The figure shows three views and two pictorial views of one solid part (mm, origin at its lowest corner). Answer the questions. A direction names the side the tool comes from. Give positions to 0.01 mm unless a question says otherwise; leave off trailing zeros. Order: outer loops, then holes, each group sorted by start corner. A loop starts at its lowest first (then second) coordinate and runs counter-clockwise, first axis right, second up. Notation, with made-up numbers: (37.5, 78) - (44.5, 78) arc R27 ccw to (44.5, 96) - close; hole circle Ø1 at (23, 56.25). An arc over 180 degrees is marked (long way). Answer as CSV lines item,"result". Start each with the question number.
1. Section A-A on y = 61 is taken. Give the vertices of the cut face in (x, z).
2. Consider line 1 along X through (y, z) = (61, 1.75); line 2 along Y through (x, z) = (31, 12); line 3 along Z through (x, y) = (41.5, 62). Determine where each line is inside the solid, lowest interval first. Write a range as [from, to].
3. Which of the six approach directions +Z, -Z, +X, -X, +Y, -Y give full straight-line access (tool end or side, diameter ignored) to the marked faces 1, 2 and 3?
4. Section D-D on y = 47.5 is taken. Give the vertices of the cut face in (x, z).
5. Section C-C on x = 56 is taken. Give the vertices of the cut face in (y, z), and give its area (3 significant figures).
6. Section B-B on z = 8 is taken. Give the vertices of the cut face in (x, y), and give its area (3 significant figures).
7. Flat-ended cylindrical pins translate along their axes: pin 1 (2 mm diameter, centred on x = 65.5, y = 57, fed in from -Z); pin 2 (1 mm diameter, centred on x = 26, z = 10.5, fed in from -Y); pin 3 (22 mm diameter, centred on x = 44.5, y = 55.5, fed in from +Z). Find the tip coordinate at first contact, or state that the pin passes through.
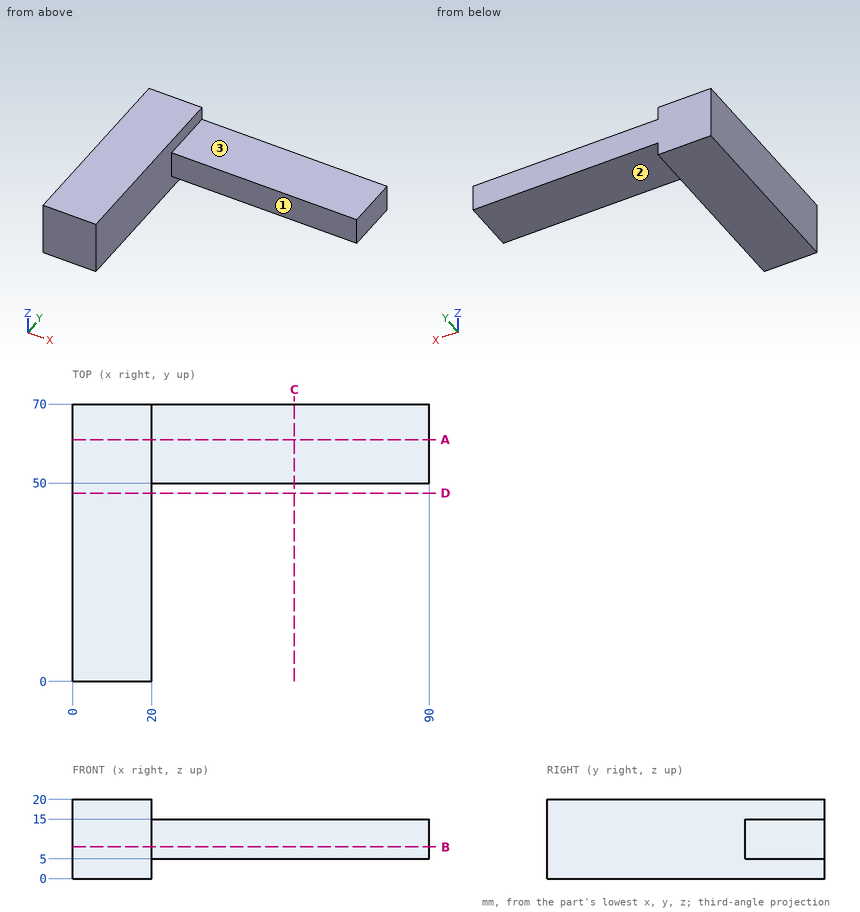
Checks:
1,outline,"(0, 0) - (20, 0) - (20, 5) - (90, 5) - (90, 15) - (20, 15) - (20, 20) - (0, 20) - close"
2,line 1,"x = [0, 20]"
2,line 2,"y = [50, 70]"
2,line 3,"z = [5, 15]"
3,face 1,"+Z, -Z, +X, -Y"
3,face 2,"-Z, +X, +Y, -Y"
3,face 3,"+Z, +X, +Y, -Y"
4,outline,"(0, 0) - (20, 0) - (20, 20) - (0, 20) - close"
5,outline,"(50, 5) - (70, 5) - (70, 15) - (50, 15) - close"
5,area,"200 mm²"
6,outline,"(0, 0) - (20, 0) - (20, 50) - (90, 50) - (90, 70) - (0, 70) - close"
6,area,"2,800 mm²"
7,pin 1,"stops at z = 5"
7,pin 2,"stops at y = 50"
7,pin 3,"stops at z = 15"
